Verification items for the finished model (mm, model axes). A direction names the side the tool comes from. Give positions to 0.01 mm unless a question says otherwise; leave off trailing zeros. Write each loop counter-clockwise with the first axis right and the second up, starting at its lowest first coordinate (ties: lowest second). Pieces come first, ordered by that corner, then holes. Notation, with made-up numbers: M 31.5,82.5 L 76.5,82.5 A9 ccw 76.5,98.5 Z; hole C 53,-21.75 d9. An arc over 180 degrees is marked long. Answer as a JSON object with one key per item and string values.
```python
from build123d import *

# Parameters (mm, degrees)
SKETCH1_R           = 60.325
BOSS_EXTRUDE1_DEPTH = 33.3375
SKETCH2_R           = 53.975
CUT_EXTRUDE1_DEPTH  = 26.9875
SKETCH3_R           = 3.175
CUT_EXTRUDE2_DEPTH  = 3.175
SKETCH4_R           = 14.2875
CUT_EXTRUDE3_DEPTH  = 90.479251261


with BuildPart() as part:
    # Sketch1 → Boss-Extrude1 (new body)
    with BuildSketch(Plane.XY):
        Circle(SKETCH1_R)
    extrude(amount=BOSS_EXTRUDE1_DEPTH)

    # Sketch2 → Cut-Extrude1 (cut)
    with BuildSketch(Plane.XY.offset(33.3375)):
        Circle(SKETCH2_R)
    extrude(amount=-CUT_EXTRUDE1_DEPTH, mode=Mode.SUBTRACT)

    # Sketch3 → Cut-Extrude2 (cut)
    with BuildSketch(Plane.XY.offset(6.35)):
        with Locations((-44.45, 0)):
            Circle(SKETCH3_R)
        with Locations((-40.607095592, 18.079443785)):
            Circle(SKETCH3_R)
        with Locations((-29.742855453, 33.032787492)):
            Circle(SKETCH3_R)
        with Locations((-13.7358054, 42.274462149)):
            Circle(SKETCH3_R)
        with Locations((4.646290192, 44.206498249)):
            Circle(SKETCH3_R)
        with Locations((22.225, 38.494829198)):
            Circle(SKETCH3_R)
        with Locations((35.9608054, 26.127054464)):
            Circle(SKETCH3_R)
        with Locations((43.478660853, 9.241674657)):
            Circle(SKETCH3_R)
        with Locations((43.478660853, -9.241674657)):
            Circle(SKETCH3_R)
        with Locations((35.9608054, -26.127054464)):
            Circle(SKETCH3_R)
        with Locations((22.225, -38.494829198)):
            Circle(SKETCH3_R)
        with Locations((4.646290192, -44.206498249)):
            Circle(SKETCH3_R)
        with Locations((-13.7358054, -42.274462149)):
            Circle(SKETCH3_R)
        with Locations((-29.742855453, -33.032787492)):
            Circle(SKETCH3_R)
        with Locations((-40.607095592, -18.079443785)):
            Circle(SKETCH3_R)
    extrude(amount=-CUT_EXTRUDE2_DEPTH, mode=Mode.SUBTRACT)

    # Sketch4 → Cut-Extrude3 (cut, through all)
    with BuildSketch(Plane.XY.offset(6.35)):
        Circle(SKETCH4_R)
    extrude(amount=-CUT_EXTRUDE3_DEPTH, mode=Mode.SUBTRACT)


solid = part.part
```
1) Thickness scan on L1, parallel to X at y = -9.5, z = 5; L2, parallel to X at y = -9, z = 3.5; L3, parallel to Z at x = 51, y = -3. Record the ranges inside material, lowest first.
Completed:
{"L1": "x = -59.57 to -10.67, 10.67 to 40.31, 46.64 to 59.57", "L2": "x = -59.65 to -11.1, 11.1 to 40.31, 46.64 to 59.65", "L3": "z = 0 to 6.35"}
2) Go/stop test with flat-tipped pins: pin 1 (12 mm diameter, centred on y = -33, z = 14.5, fed in from +X); pin 2 (8.5 mm diameter, centred on x = -40.61, y = -18.08, fed in from +Z); pin 3 (3 mm diameter, centred on x = -29, y = -34.5, fed in from +Z) (3 decimals). Record where each tip stops, or that it passes through.
Completed:
{"pin 1": "stops at x = 53.95", "pin 2": "stops at z = 6.35", "pin 3": "stops at z = 3.175"}
3) Release check for a two-part mould opening along X. For faces 3 (the face through (-45, -31, 33.338)), 4 (the face through (40.307, -9.102, 4.785)) record: pulls with the +X half, pulls with the -X half, needs draft (parallel to the pull), parting line crosses it, or undercut.
Completed:
{"face 3": "needs draft", "face 4": "undercut"}
4) Access from +Z, -Z, +X, -X, +Y, -Y to the whole of each face (thin tool, end or side, straight path). Record for faces 1 (the face through (-14.274, 0.628, 3.219)), 2 (the face through (6.353, 46.884, 4.785)).
Completed:
{"face 1": "+Z, -Z", "face 2": "+Z"}
5) Section check C-C on z = 23.5. Record the boundary of the cut face in (x, y) (3 decimals).
Completed:
{"outline": "C 0,0 d120.65; hole C 0,0 d107.95"}
6) Section check D-D on x = -34.5. Record the boundary of the cut face in (y, z).
Completed:
{"outline": "M -49.49,0 L 49.49,0 L 49.49,33.34 L 41.51,33.34 L 41.51,6.35 L -41.51,6.35 L -41.51,33.34 L -49.49,33.34 Z"}
